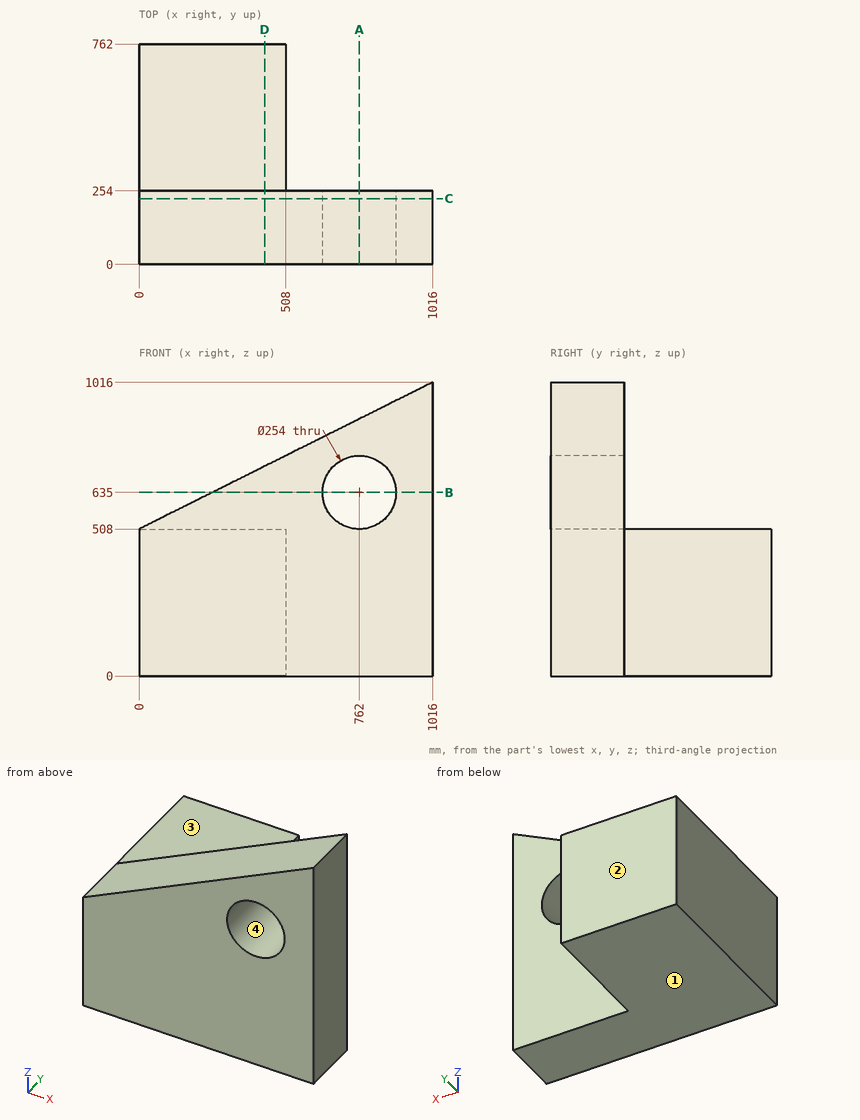
Study the drawing (mm; zero at the part's minimum x, y, z) and answer. Give positions to 0.01 mm unless a question says otherwise; leave off trailing zeros. Write each loop counter-clockwise with the first axis right and the second up, starting at its lowest first coordinate (ties: lowest second). Pieces come first, ordered by that corner, then holes. Notation, with made-up numbers: M 84.5,-1 L 92.5,-1 A12 cw 92.5,6 Z; hole C 49.25,-32.5 d6. An arc over 180 degrees is marked long. Put each result on its own line as item: value. Start each with the question number.
1. The part is cut by section A-A, the plane x = 762. Give the vertices of the cut face in (y, z).
2. Consider line 1 along X through (y, z) = (196, 635); line 2 along Z through (x, y) = (382.5, 378). Determine where each line is inside the solid, lowest interval first.
3. Each of these flat-tipped pins is pushed along its axis until it touches: pin 1 Ø2 at (y, z) = (199.5, 584.5) entering from -X; pin 2 Ø3 at (x, y) = (427, 631.5) entering from +Z; pin 3 Ø6 at (x, z) = (520.5, 599.5) entering from +Y. Where does it stop, or does it pass through?
4. The part is cut by section B-B, the plane z = 635. Give the vertices of the cut face in (x, y).
5. The part is cut by section D-D, the plane x = 434.5. Give the vertices of the cut face in (y, z).
6. The part is cut by section C-C, the plane y = 227.5. Give the vertices of the cut face in (x, z), and give its area (3 significant figures).
7. For a pull along Z with two mould halves and no side action, classify the marked faces 1, 2, 3 and 4 as released by +Z, released by -Z, zero draft, split by the parting line, or undercut.
Final values:
1. outline: M 0,0 L 254,0 L 254,508 L 0,508 Z; M 0,762 L 254,762 L 254,889 L 0,889 Z
2. line 1: x = 254 to 635, 889 to 1016
2. line 2: z = 0 to 508
3. pin 1: stops at x = 151
3. pin 2: stops at z = 508
3. pin 3: stops at y = 254
4. outline: M 254,0 L 635,0 L 635,254 L 254,254 Z; M 889,0 L 1016,0 L 1016,254 L 889,254 Z
5. outline: M 0,0 L 762,0 L 762,508 L 254,508 L 254,725.25 L 0,725.25 Z
6. outline: M 0,0 L 1016,0 L 1016,1016 L 0,508 Z; hole C 762,635 d254
6. area: 724,000 mm²
7. face 1: released by -Z
7. face 2: zero draft
7. face 3: released by +Z
7. face 4: undercut
